Verification items for the finished model (mm, model axes). Face numbers are marked on the shaded views. Coordinates: 2 decimals unless noted, no trailing zeros. Order: outer loops, then holes, each group sorted by start corner. A loop starts at its lowest first (then second) coordinate and runs counter-clockwise, first axis right, second up. Notation, with made-up numbers: (18, 69) -> (67, 69) arc R30 cw to (67, 95) -> close; hole circle Ø2 at (29.25, 12.25). An arc over 180 degrees is marked (long way). Answer as CSV lines item,"result".
```python
from build123d import *

# Parameters (mm, degrees)
CHAMFER1_SIZE = 0.762
FILLET1_R     = 1.27
FILLET2_R     = 1.27
FILLET3_R     = 5.08


with BuildPart() as part:
    # Sketch1 → Revolve1 (revolve)
    with BuildSketch(Plane.XY, mode=Mode.PRIVATE) as revolve1_sk:
        Polygon((-27.94, 107.95), (-8.255, 88.265), (-8.255, 0), (-5.08, 0), (-5.08, 12.7), (0, 12.7), (0, 98.95), (-3, 98.95), (-3, 107.95), align=None)
    revolve(revolve1_sk.sketch.rotate(Axis((0, 12.7, 0), (0, 1, 0)), 270), axis=Axis((0, 12.7, 0), (0, 1, 0)))

    # Chamfer1
    chamfer1_edges = [part.edges().sort_by_distance(p)[0] for p in [
        (0, 0, 5.08),
        (0, 107.95, 3),
    ]]
    chamfer(chamfer1_edges, length=CHAMFER1_SIZE)

    # Fillet1
    fillet1_edges = [part.edges().sort_by_distance(p)[0] for p in [
        (0, 0, 8.255),
    ]]
    fillet(fillet1_edges, radius=FILLET1_R)

    # Fillet2
    fillet2_edges = [part.edges().sort_by_distance(p)[0] for p in [
        (0, 107.95, 27.94),
    ]]
    fillet(fillet2_edges, radius=FILLET2_R)

    # Fillet3
    fillet3_edges = [part.edges().sort_by_distance(p)[0] for p in [
        (0, 88.265, 8.255),
    ]]
    fillet(fillet3_edges, radius=FILLET3_R)


solid = part.part
```
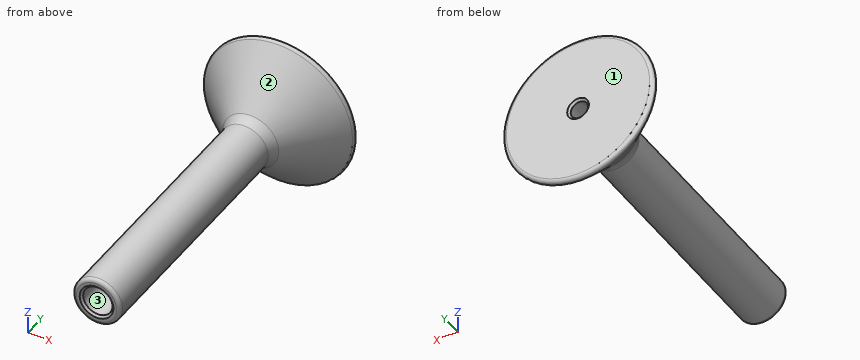
Item 1: Thickness scan on line 1 (X direction, y = 3.5, z = 0) (3 decimals); line 2 (X direction, y = 4, z = -3); line 3 (X direction, y = 55, z = 0.5). Record the ranges inside material, lowest first.
Answer list:
line 1,"-8.255 to -5.08, 5.08 to 8.255"
line 2,"-7.69 to -4.1, 4.1 to 7.69"
line 3,"-8.24 to 8.24"
Item 2: Depth check by flat-ended pin: pin 1 Ø2 at (x, y) = (1.5, 62) entering from +Z; pin 2 Ø12 at (x, y) = (8.5, 79.5) entering from -Z; pin 3 Ø2 at (x, z) = (16, 6) entering from -Y. Enter the tip coordinate at first touch or a pass-through.
Answer list:
pin 1,"z = 8.24"
pin 2,"z = -7.87"
pin 3,"y = 96.1"
Item 3: Release check for a two-part mould opening along Z. For the marked faces 1, 2 and 3 record: +Z half, -Z half, draft (parallel to the pull), parting line (faces both ways), or undercut.
Answer list:
face 1,"draft"
face 2,"parting line"
face 3,"undercut"
Item 4: Section check A-A, the plane y = 79. Record the boundary of the cut face in (x, z) (3 decimals).
Answer list:
outline,"circle Ø16.51 at (0, 0)"
